Part print with two shaded views. Sizes in mm from the minimum x, y, z corner. A direction names the side the tool comes from. Give positions to 0.01 mm unless a question says otherwise; leave off trailing zeros. Write each loop counter-clockwise with the first axis right and the second up, starting at its lowest first coordinate (ties: lowest second). Pieces come first, ordered by that corner, then holes. Notation, with made-up numbers: M 24.25,0 L 54.25,0 A31 ccw 54.25,37 Z; hole C -11,76.25 d3. An arc over 180 degrees is marked long. One line per item, written item: value. Start each with the question number.
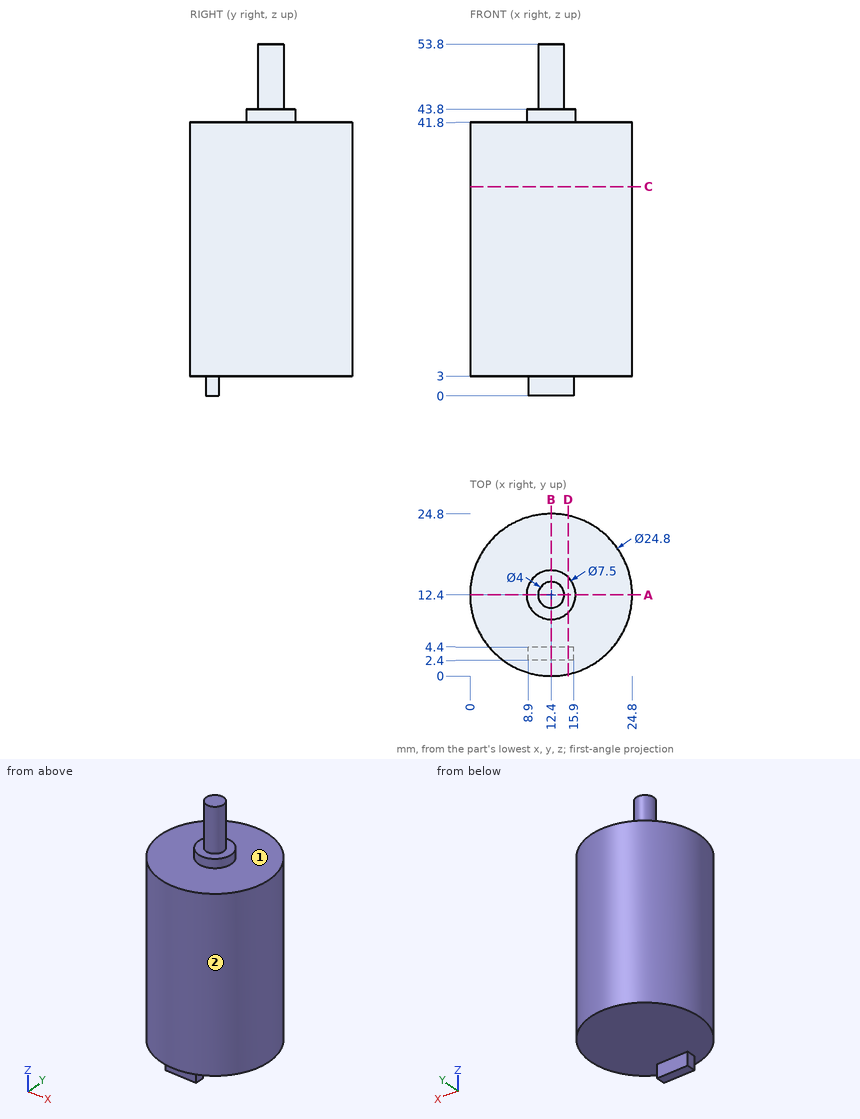
1) Tool access for the marked faces 1 and 2: list every direction of +Z, -Z, +X, -X, +Y, -Y with a clear straight run to the whole face (end or side of a thin tool).
2) Probe line 1 along Z through (x, y) = (14.5, 16.5); line 2 along Z through (x, y) = (14, 12.5); line 3 along Y through (x, z) = (12.5, 30.5). List the from-to ranges inside material, lowest first. Write a range as from..to.
3) Drop flat-ended pins along their axis: P1, Ø10, axis at y = 15, z = 40.5, coming from the +X side; P2, Ø5, axis at y = 12.5, z = 47, coming from the -X side; P3, Ø1, axis at y = 15, z = 27.5, coming from the +X side; P4, Ø4, axis at y = 10, z = 7, coming from the -X side. Give the stop position or say it passes through.
4) Band-saw the part on C-C (z = 32). List the corners of the cut face in (x, y).
5) Band-saw the part on D-D (x = 15). List the corners of the cut face in (y, z).
6) Band-saw the part on A-A (y = 12.4). List the corners of the cut face in (x, z), then the cut area to 3 significant figures.
7) Band-saw the part on B-B (x = 12.4). List the corners of the cut face in (y, z), then the cut area to 3 significant figures.
Model answer:
1. face 1: +Z
1. face 2: +Z, -Z
2. line 1: z = 3..41.8
2. line 2: z = 3..53.8
2. line 3: y = 0..24.8
3. P1: stops at x = 24.8
3. P2: stops at x = 10.4
3. P3: stops at x = 24.62
3. P4: stops at x = 0.01
4. outline: C 12.4,12.4 d24.8
5. outline: M 0.28,3 L 2.4,3 L 2.4,0 L 4.4,0 L 4.4,3 L 24.52,3 L 24.52,41.8 L 15.1,41.8 L 15.1,43.8 L 9.7,43.8 L 9.7,41.8 L 0.28,41.8 Z
6. outline: M 0,3 L 24.8,3 L 24.8,41.8 L 16.15,41.8 L 16.15,43.8 L 14.4,43.8 L 14.4,53.8 L 10.4,53.8 L 10.4,43.8 L 8.65,43.8 L 8.65,41.8 L 0,41.8 Z
6. area: 1,020 mm²
7. outline: M 0,3 L 2.4,3 L 2.4,0 L 4.4,0 L 4.4,3 L 24.8,3 L 24.8,41.8 L 16.15,41.8 L 16.15,43.8 L 14.4,43.8 L 14.4,53.8 L 10.4,53.8 L 10.4,43.8 L 8.65,43.8 L 8.65,41.8 L 0,41.8 Z
7. area: 1,020 mm²
